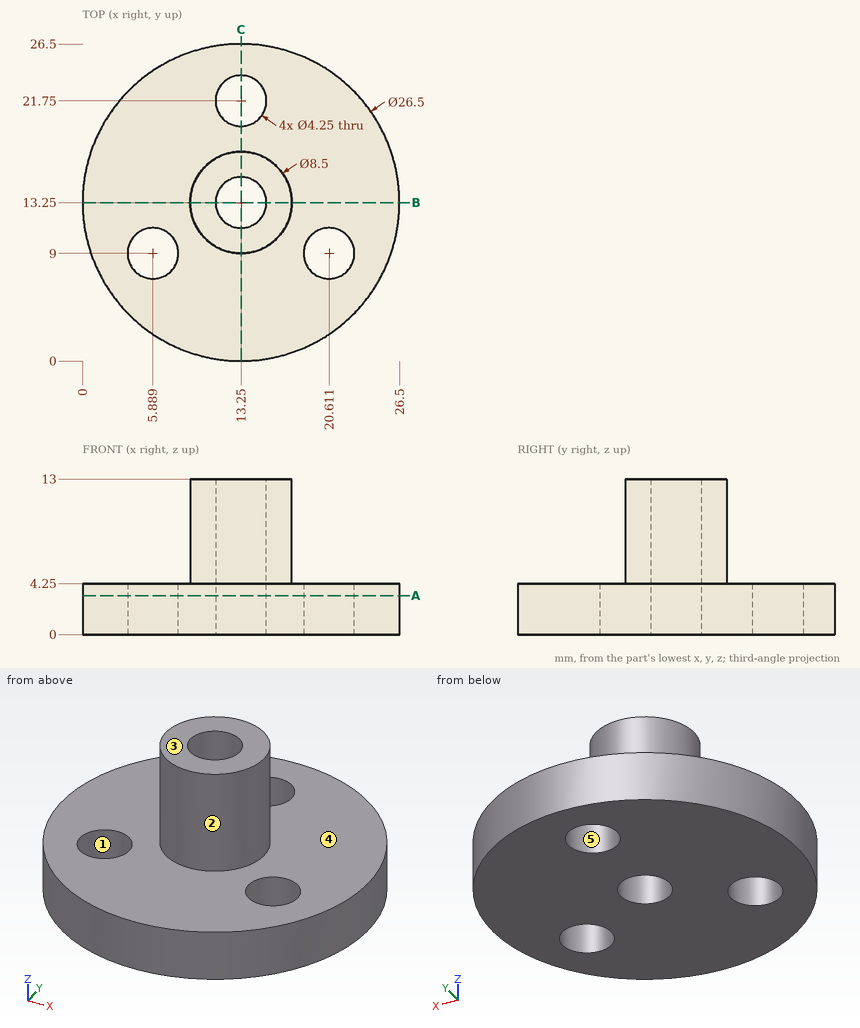
Design review of the part shown in the three views and the two pictorial views. Dimensions are in mm from the part's minimum x, y and z. A direction names the side the tool comes from. Round coordinates to 2 decimals unless told otherwise and drop trailing zeros. Order: outer loops, then holes, each group sorted by start corner. A loop starts at its lowest first (then second) coordinate and runs counter-clockwise, first axis right, second up. Notation, with made-up numbers: (53.5, 15.5) - (107.5, 15.5) arc R15 cw to (107.5, 32.5) - close; hole circle Ø5 at (-15, 81). An arc over 180 degrees is marked (long way). One line per question, with ' | ' between items.
Item 1: Take a section at A-A, the plane z = 3.25. Give the number of separate pieces and of enclosed holes in the cut face, then the cut area to 3 significant figures.
Checks:
separate pieces: 1 | enclosed holes: 4 | area: 495 mm²
Item 2: Take a section at C-C, the plane x = 13.25. Write out the cut boundary in (y, z) (3 decimals).
Checks:
outline: (0, 0) - (11.125, 0) - (11.125, 13) - (9, 13) - (9, 4.25) - (0, 4.25) - close; (15.375, 0) - (19.625, 0) - (19.625, 4.25) - (17.5, 4.25) - (17.5, 13) - (15.375, 13) - close; (23.875, 0) - (26.5, 0) - (26.5, 4.25) - (23.875, 4.25) - close
Item 3: Draft analysis for pull direction Y (two halves, no side actions). For the marked faces 1, 2 and 3, state which applies: +Y half, -Y half, draft (parallel to the pull), parting line (faces both ways), or undercut.
Checks:
face 1: undercut | face 2: parting line | face 3: draft
Item 4: For P1, Ø3.5, axis at x = 13.25, y = 21.75, coming from the +Z side; P2, Ø4, axis at y = 17.5, z = 9, coming from the +X side (1 decimal); P3, Ø3, axis at x = 16.5, y = 22, coming from the -Z side; P4, Ø4, axis at x = 5, z = 3.5, coming from the +Y side, all flat-tipped, find the tip position at first contact; note any pin that passes through.
Checks:
P1: through | P2: x = 16.9 | P3: z = 0 | P4: y = 24.93
Item 5: Take a section at B-B, the plane y = 13.25. Write out the cut boundary in (x, z) (3 decimals), then the cut area to 3 significant figures.
Checks:
outline: (0, 0) - (11.125, 0) - (11.125, 13) - (9, 13) - (9, 4.25) - (0, 4.25) - close; (15.375, 0) - (26.5, 0) - (26.5, 4.25) - (17.5, 4.25) - (17.5, 13) - (15.375, 13) - close | area: 132 mm²
Item 6: Wall thickness on line 1 (Y direction, x = 13.25, z = 2.55) (3 decimals); line 2 (Z direction, x = 24.25, y = 13.5); line 3 (Y direction, x = 13.25, z = 4.5) (3 decimals): over which ranges is each line inside the solid? List them lowest first. Write a range as [from, to].
Checks:
line 1: [0, 11.125], [15.375, 19.625], [23.875, 26.5] | line 2: [0, 4.25] | line 3: [9, 11.125], [15.375, 17.5]
Item 7: Machinability: for the marked faces 4 and 5, which of the approach directions +Z, -Z, +X, -X, +Y, -Y give a long, thin tool a straight path to every point of the face, cutting with its end or side? Answer none if there is none.
Checks:
face 4: +Z | face 5: +Z, -Z
